Can you work these out from the model? Positions are in its coordinate system, mm. A direction names the side the tool comes from. Give positions to 0.01 mm unless a question says otherwise; leave off trailing zeros. Write each loop counter-clockwise with the first axis right and the second up, starting at its lowest first coordinate (ties: lowest second). Pieces come first, ordered by that corner, then holes.
1. I'm going to push flat-ended pins straight in: pin 1 (2 mm diameter, centred on x = -9.5, y = 0, fed in from -Z); pin 2 (10 mm diameter, centred on y = 3.5, z = 5.5, fed in from -X); pin 3 (3 mm diameter, centred on x = 8, z = 3, fed in from -Y); pin 4 (5 mm diameter, centred on y = 5.5, z = -4.5, fed in from +X). Where does each tip first touch, or does it pass through?
2. If I drill on probe 1 along Z at (x, y) = (9, -2); probe 2 along Y at (x, z) = (-1.25, 5.5); probe 3 along X at (y, z) = (5.75, 1.75), over which ranges is the centre line in solid material (lowest first)?
3. Suppose I cut it at D-D (z = 6.25). Please give me the cut outline in (x, y).
4. Suppose I cut it at B-B (z = 1.5). Please give me the cut outline in (x, y), and give its area (3 significant figures).
5. On a 3-axis mill with a long thin cutter (end or side, diameter ignored), from which of +Z, -Z, +X, -X, +Y, -Y can I reach the whole of each face in a straight line? I mean faces 4 (the flat face through (-5, -9, 0)), 5 (the cylindrical face through (1.46, 6.59, -9.86)), 6 (the cylindrical face through (-6, 0, 8)), 7 (the flat face through (0, 0, -12.4)). Say none if no direction works.
6. Suppose I cut it at A-A (y = -8). Please give me the cut outline in (x, z).
7. Thinking about a two-plate mould opening in Z: for faces 1 (the cylindrical face through (5.158, 3.955, -7.197)), 2 (the flat face through (0, -9.5, 2)), 3 (the flat face through (-5, 9, 0)), which applies, pulls with the +Z half, pulls with the -Z half, needs draft (parallel to the pull), parting line crosses it, or undercut?
Autodesk Inventor part; units mm, degrees
ref_plane "YZ Plane" through (0, 0, 0) normal (1, 0, 0) x (0, 1, 0)
ref_plane "XZ Plane" through (0, 0, 0) normal (0, 1, 0) x (-1, 0, 0)
ref_plane "XY Plane" through (0, 0, 0) normal (0, 0, 1) x (1, 0, 0)
sketch "Sketch2" plane through (0, 0, 0) normal (0, 0, 1) x (1, 0, 0)
  line L0 (10.9697, 0) -> (5.4848, -9.5)
  line L1 (5.4848, -9.5) -> (-5.4848, -9.5)
  line L2 (-5.4848, -9.5) -> (-10.9697, 0)
  line L3 (-10.9697, 0) -> (-5.4848, 9.5)
  line L4 (-5.4848, 9.5) -> (5.4848, 9.5)
  line L5 (5.4848, 9.5) -> (10.9697, 0)
  point P0 (0, 0)
  point P1 (0, 0)
  dimension "d2" = 9.5
  dimension "d3" = 19
extrude "Extrusion1" add sketch "Sketch2" along normal blind 3.5
sketch "Sketch3" plane through (0, 0, 3.5) normal (0, 0, 1) x (1, 0, 0)
  circle A0 centre (0, 0) radius 6
  dimension "d6" = 12
extrude "Extrusion2" add sketch "Sketch3" along normal blind 9.5
sketch "Sketch4" plane through (0, 0, 0) normal (0, 0, -1) x (-1, 0, 0)
  circle A0 centre (0, 0) radius 9.5
  dimension "d9" = 19
extrude "Extrusion3" add sketch "Sketch4" along normal blind 5
sketch "Sketch5" plane through (0, 0, -5) normal (0, 0, -1) x (-1, 0, 0)
  circle A0 centre (0, 0) radius 7
  dimension "d12" = 14
extrude "Extrusion4" add sketch "Sketch5" along normal blind 2
sketch "Sketch6" plane through (0, 0, -7) normal (0, 0, -1) x (-1, 0, 0)
  circle A0 centre (0, 0) radius 6.5
  dimension "d15" = 13
extrude "Extrusion5" add sketch "Sketch6" along normal blind 0.4
sketch "Sketch7" plane through (0, 0, -7.4) normal (0, 0, -1) x (-1, 0, 0)
  circle A0 centre (0, 0) radius 6.75
  dimension "d18" = 13.5
extrude "Extrusion6" add sketch "Sketch7" along normal blind 5
thread "Thread1"
properties part number "NPI-19M-030G2"
Checks:
1. pin 1: stops at z = -5
1. pin 2: stops at x = -10.97
1. pin 3: stops at y = -7.74
1. pin 4: stops at x = 9.01
2. probe 1: z = -5 to 3.5
2. probe 2: y = -5.87 to 5.87
2. probe 3: x = -7.65 to 7.65
3. outline: circle Ø12 at (0, 0)
4. outline: (-10.97, 0) - (-5.48, -9.5) - (5.48, -9.5) - (10.97, 0) - (5.48, 9.5) - (-5.48, 9.5) - close
4. area: 313 mm2
5. face 4: -Z, -X, -Y
5. face 5: -Z
5. face 6: +Z
5. face 7: -Z, +X, -X, +Y, -Y
6. outline: (-6.35, 0) - (-5.12, 0) - (-5.12, -5) - (5.12, -5) - (5.12, 0) - (6.35, 0) - (6.35, 3.5) - (-6.35, 3.5) - close
7. face 1: undercut
7. face 2: needs draft
7. face 3: pulls with the -Z half
